Geometry: see drawing. Coordinates: mm, zero at the bounding-box minimum. A direction names the side the tool comes from. Give positions to 0.01 mm unless a question says otherwise; leave off trailing zeros. Write each loop counter-clockwise with the first axis right and the second up, starting at its lowest first coordinate (ties: lowest second). Pieces come first, ordered by that corner, then holes. Notation, with made-up numbers: M -22,87.5 L -9,87.5 A18 cw -9,114.5 Z; hole C 54.25,11.25 d5. An arc over 180 degrees is marked long. Use one line per item in the form item = value. Start each with the question number.
Item 1: Contact query for flat-ended pins moving along their axis: P1, Ø1, axis at x = 1.5, z = 22.5, coming from the +Y side; P2, Ø1, axis at x = 2.5, z = 7.5, coming from the -Y side; P3, Ø3, axis at x = 2, z = 24.5, coming from the -Y side. Output: stop coordinate, or through.
Item 2: Access query for the marked faces 1 and 2. Directions: +Z, -Z, +X, -X, +Y, -Y. A direction counts if a zero-diameter tool reaches every point of the face in a straight line with its end or side. Return the directions, or none.
Item 3: Section query D-D on x = 3.05. Return loops of the section in (y, z), then the cut area to 3 significant figures.
Item 4: Material intervals for line 1 along X through (y, z) = (7.65, 14.1); line 2 along Z through (x, y) = (3.5, 14.25); line 3 along X through (y, z) = (6.5, 2.5), sorted ascending. Write a range as from..to.
Item 5: Section query A-A on y = 14.1. Return loops of the section in (x, z), then the cut area to 3 significant figures.
Item 6: Pull-direction query (Z, two-part tool) for the marked faces 3, 4 and 5; classes: released by +Z, released by -Z, zero draft, split by the parting line, or undercut.
Item 7: Section query B-B on z = 14.1. Return loops of the section in (x, y).
Item 8: Section query C-C on y = 9.25. Return loops of the section in (x, z), then the cut area to 3 significant figures.
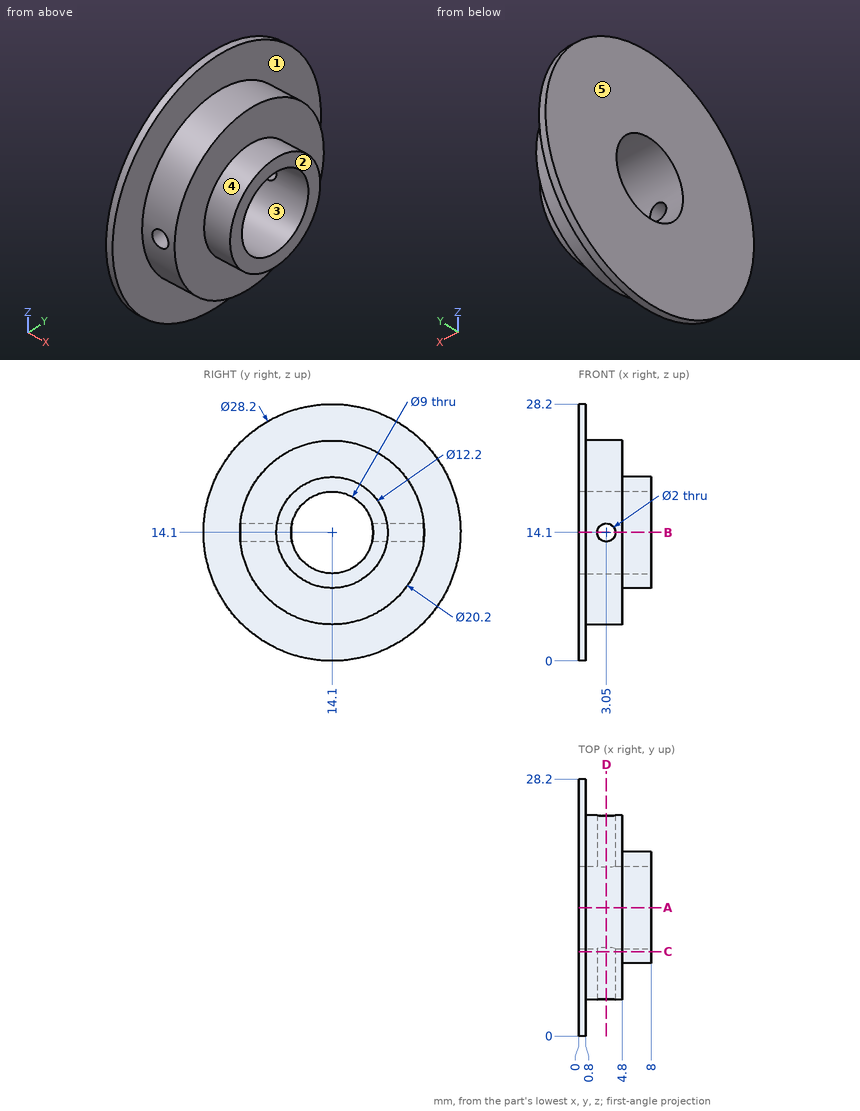
Answer sheet:
q1.P1 = 20.39
q1.P2 = 6.05
q1.P3 = 3.68
q2.face_1 = +X
q2.face_2 = +Z, -Z, +X, +Y, -Y
q3.outline = M 4.05,13.1 A10.1 ccw 24.15,13.1 L 18.49,13.1 A4.5 cw 9.71,13.1 Z; M 4.05,15.1 L 9.71,15.1 A4.5 cw 18.49,15.1 L 24.15,15.1 A10.1 ccw Z
q3.area = 234 mm2
q4.line_1 = 0..2.05, 4.05..4.8
q4.line_2 = 4..9.6, 18.6..24.2
q4.line_3 = 0..0.8
q5.outline = M 0,0 L 0.8,0 L 0.8,4 L 4.8,4 L 4.8,8 L 8,8 L 8,9.6 L 0,9.6 Z; M 0,18.6 L 8,18.6 L 8,20.2 L 4.8,20.2 L 4.8,24.2 L 0.8,24.2 L 0.8,28.2 L 0,28.2 Z
q5.area = 70.4 mm2
q6.face_3 = undercut
q6.face_4 = split by the parting line
q6.face_5 = zero draft
q7.outline = M 0,0 L 0.8,0 L 0.8,4 L 2.05,4 L 2.05,9.6 L 0,9.6 Z; M 0,18.6 L 2.05,18.6 L 2.05,24.2 L 0.8,24.2 L 0.8,28.2 L 0,28.2 Z; M 4.05,4 L 4.8,4 L 4.8,8 L 8,8 L 8,9.6 L 4.05,9.6 Z; M 4.05,18.6 L 8,18.6 L 8,20.2 L 4.8,20.2 L 4.8,24.2 L 4.05,24.2 Z
q8.outline = M 0,0.86 L 0.8,0.86 L 0.8,5.24 L 4.8,5.24 L 4.8,10.4 L 8,10.4 L 8,17.8 L 4.8,17.8 L 4.8,22.96 L 0.8,22.96 L 0.8,27.34 L 0,27.34 Z; hole C 3.05,14.1 d2
q8.area = 113 mm2
